Geometry: final body of the model. Coordinates: model frame, mm. A direction names the side the tool comes from. Round coordinates to 2 decimals unless told otherwise and drop trailing zeros. Write each loop counter-clockwise with the first axis right and the second up, starting at its lowest first coordinate (ties: lowest second). Pieces come first, ordered by that corner, then holes. Notation, with made-up numbers: M 43,7.5 L 75,7.5 A20 cw 75,43.5 Z; hole C 62,51 d5. An arc over 180 degrees is marked long. Use one line per item in the form item = value. Start each with the question number.
from build123d import *

# Parameters (mm, degrees)
F0_R     = 14
F0_W     = 11
F0_H     = 7.7
F1_DEPTH = 40


with BuildPart() as f1:
    # F0 (on Front) → F1 (new body)
    with BuildSketch(Plane.XZ):
        Polygon((47.230265, 7.764964), (47.230265, 0), (58.230265, 0), (67.730265, 0), (67.730265, 15), (61.730265, 15), (61.730265, 7.7), align=None)
        Polygon((-42.269735, 15), (-42.269735, 0), (-32.769735, 0), (-32.769735, 7.7), (-36.269735, 7.7), (-36.269735, 15), align=None)
        Polygon((43.730265, 7.780645), (47.230265, 7.764964), (61.730265, 7.7), (61.730265, 15), (43.730265, 15.080645), align=None)
        Polygon((-36.269735, 7.7), (-32.769735, 7.7), (-21.769735, 7.7), (-18.269735, 7.7), (-18.269735, 15), (-36.269735, 15), align=None)
        with BuildLine():
            Line((-21.769735, 7.7), (-21.769735, 0))
            Line((-21.769735, 0), (47.230265, 0))
            Line((47.230265, 0), (47.230265, 7.764964))
            Line((47.230265, 7.764964), (43.730265, 7.780645))
            Line((43.730265, 7.780645), (43.730265, 15.080645))
            Line((43.730265, 15.080645), (37.730265, 15.080645))
            Line((37.730265, 15.080645), (37.730265, 40))
            Line((37.730265, 40), (37.730265, 40.080645))
            ThreePointArc((37.730265, 40.080645), (12.689942, 65.040323), (-12.269735, 40))
            Line((-12.269735, 40), (-12.269735, 15))
            Line((-12.269735, 15), (-18.269735, 15))
            Line((-18.269735, 15), (-18.269735, 7.7))
            Line((-18.269735, 7.7), (-21.769735, 7.7))
        make_face()
        with Locations((12.730265, 40.040323)):
            Circle(F0_R, mode=Mode.SUBTRACT)
        with Locations((12.730265, 40.040323)):
            Circle(F0_R)
        with Locations((-27.269735, 3.85)):
            Rectangle(F0_W, F0_H)
    extrude(amount=F1_DEPTH)


solid = f1.part
1. Section query B-B (z = 25). Return loops of the section in (x, y), then the cut area to 3 significant figures.
2. Section query C-C (x = -25). Return loops of the section in (y, z), then the cut area to 3 significant figures.
3. Set-up query: faces 1 (the face through (12, -20, 0)), 2 (the face through (41, -20, 15.081)), 3 (the face through (-27, -20, 15)). Return all of +Z, -Z, +X, -X, +Y, -Y with unobstructed straight access to the full face (end or side cutting, diameter ignored); none if empty.
4. Ray query, probe 1 along X at (y, z) = (-22.5, 30); probe 2 along Z at (x, y) = (13, -6.5); probe 3 along Z at (x, y) = (56, -23). Return the intervals inside material, ascending.
5. Contact query for flat-ended pins moving along their axis: pin 1 (9 mm diameter, centred on x = -21.5, y = -19, fed in from +Z); pin 2 (20 mm diameter, centred on y = -13, z = 27.5, fed in from +X); pin 3 (1.5 mm diameter, centred on x = 42, y = -29, fed in from +Z); pin 4 (10 mm diameter, centred on x = 41.5, z = 22, fed in from -Y). Output: stop coordinate, or through.
6. Section query A-A (y = -30). Return loops of the section in (x, z), then the cut area to 3 significant figures.
Checks:
q1.outline = M -12.27,-40 L 37.73,-40 L 37.73,0 L -12.27,0 Z
q1.area = 2,000 mm^2
q2.outline = M -40,0 L 0,0 L 0,15 L -40,15 Z
q2.area = 600 mm^2
q3.face_1 = -Z, +X, -X, +Y, -Y
q3.face_2 = +Z, +X, +Y, -Y
q3.face_3 = +Z, -X, +Y, -Y
q4.probe_1 = -12.27 to 37.73
q4.probe_2 = 0 to 65.04
q4.probe_3 = 0 to 15.03
q5.pin_1 = 15
q5.pin_2 = 37.73
q5.pin_3 = 15.08
q5.pin_4 = -40
q6.outline = M -42.27,0 L 67.73,0 L 67.73,15 L 61.73,15 L 43.73,15.08 L 37.73,15.08 L 37.73,40.08 A25 ccw -12.27,40 L -12.27,15 L -42.27,15 Z
q6.area = 3,880 mm^2
